Input: part model. Units: mm. Frame: model coordinates. Face numbers are marked on the shaded views. Round coordinates to 2 decimals unless told otherwise and drop trailing zeros. Order: outer loops, then holes, each group sorted by start corner. A loop starts at its lowest first (then second) coordinate and runs counter-clockwise, first axis right, second up. Notation, with made-up numbers: M 79,81 L 91,81 A18 cw 91,114 Z; hole C 29,71.25 d10. An arc over 180 degrees is marked long. One line per question, with ' | ' between items.
```python
from build123d import *

# Parameters (mm, degrees)
F_8_32_TAPPED_HOLE1_D           = 3.4544
F_8_32_TAPPED_HOLE1_DEPTH       = 15.07744
F_8_32_TAPPED_HOLE1_CBORE_D     = 4.1656
F_8_32_TAPPED_HOLE1_CBORE_DEPTH = 12.7
F_8_32_TAPPED_HOLE1_TIP         = 1.037806461


with BuildPart() as part:
    # Sketch1 → Base-Revolve (revolve)
    with BuildSketch(Plane.XY):
        with BuildLine():
            Line((0, 0), (-9.525, 0))
            Line((-9.525, 0), (-9.525, 3.175))
            ThreePointArc((-9.525, 3.175), (-6.350520234, 8.282737448), (-9.387318408, 13.47351393))
            ThreePointArc((-9.387318408, 13.47351393), (-11.809371387, 15.806889756), (-12.7, 19.05))
            add(Edge.make_bspline(
                [(0, 25.4), (-12.7, 25.4), (-12.7, 19.05)],
                knots=[4.71238898, 4.71238898, 4.71238898, 6.283185307, 6.283185307, 6.283185307], degree=2, weights=[1, 0.707106781, 1]))
            Line((0, 25.4), (0, 0))
        make_face()
    revolve(axis=Axis((0, 0, 0), (0, 1, 0)))

    # #8-32 Tapped Hole1
    with Locations(Plane.XZ):
        with Locations((0, 0)):
            CounterBoreHole(F_8_32_TAPPED_HOLE1_D / 2, F_8_32_TAPPED_HOLE1_CBORE_D / 2, F_8_32_TAPPED_HOLE1_CBORE_DEPTH, depth=F_8_32_TAPPED_HOLE1_DEPTH)
            with Locations((0, 0, -(F_8_32_TAPPED_HOLE1_DEPTH + F_8_32_TAPPED_HOLE1_TIP / 2))):  # 118° drill point
                Cone(0, F_8_32_TAPPED_HOLE1_D / 2, F_8_32_TAPPED_HOLE1_TIP, mode=Mode.SUBTRACT)


solid = part.part
```
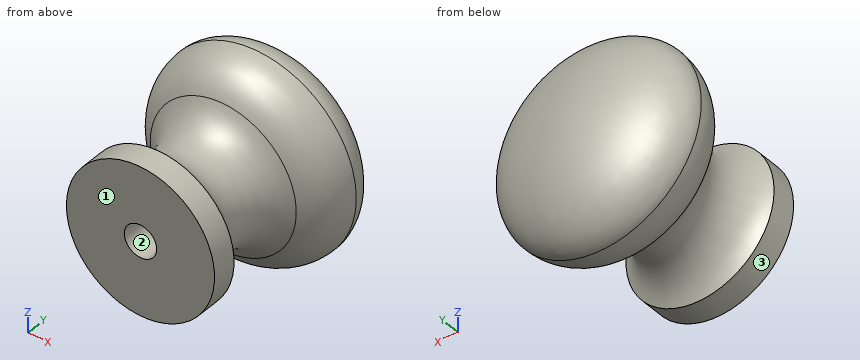
Item 1: First-contact query: pin 1 (1.5 mm diameter, centred on x = -9, z = -6, fed in from +Y); pin 2 (1 mm diameter, centred on y = 15, z = -1.5, fed in from -X); pin 3 (8 mm diameter, centred on x = 7, y = 12, fed in from -Z); pin 4 (2 mm diameter, centred on x = -4.5, z = 8.5, fed in from -Y). Flat tips, straight axial feed; report the tip coordinate or a pass-through.
Report:
pin 1: y = 22.92 | pin 2: x = -11.52 | pin 3: z = -10.46 | pin 4: y = 0
Item 2: Line query: line 1 along Z through (x, y) = (0, 6); line 2 along Z through (x, y) = (-1.75, 8.25); line 3 along X through (y, z) = (3.5, -0.25). Output: solid intervals per line, ascending. Write a range as from..to.
Report:
line 1: -6.85..-2.08, 2.08..6.85 | line 2: -6.11..-1.13, 1.13..6.11 | line 3: -8.96..-2.07, 2.07..8.96
Item 3: Section query A-A, the plane y = 7.75. Return loops of the section in (x, z).
Report:
outline: C 0,0 d12.76; hole C 0,0 d4.17
Item 4: Mould query, pull axis X, two halves, no side actions, for the marked faces 1, 2 and 3. Classes: +X half, -X half, draft (parallel to the pull), parting line (faces both ways), or undercut.
Report:
face 1: draft | face 2: undercut | face 3: parting line
